Geometry: final body of the model. Coordinates: model frame, mm. Face numbers are marked on the shaded views. A direction names the side the tool comes from. Give positions to 0.01 mm unless a question says otherwise; leave off trailing zeros. Loops run counter-clockwise (first coordinate to the right, second up) from the corner with the lowest first, then second, coordinate; pieces in that order, holes last. Notation, with made-up numbers: M 52,50 L 58,50 A28 ccw 58,75 Z; hole C 42.25,78 d6. An arc over 180 degrees is marked long. Put each result on its own line as item: value.
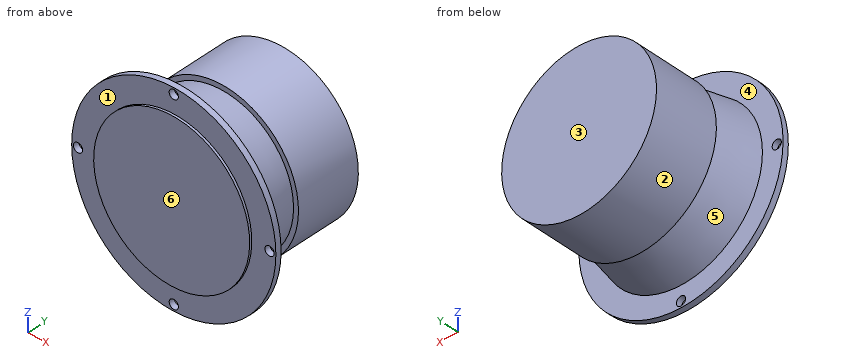
```python
from build123d import *

# Parameters (mm, degrees)
SKETCH1_R           = 44.5
SKETCH1_R_2         = 2
BOSS_EXTRUDE1_DEPTH = 2.5
SKETCH2_R           = 34
BOSS_EXTRUDE2_DEPTH = 1
SKETCH3_R           = 35.5
BOSS_EXTRUDE3_DEPTH = 20
BOSS_EXTRUDE3_TAPER = 11
SKETCH4_R           = 33.75
BOSS_EXTRUDE4_DEPTH = 28.5


with BuildPart() as part:
    # Sketch1 → Boss-Extrude1 (new body)
    with BuildSketch(Plane(origin=(0, 0, 0), x_dir=(1, 0, 0), z_dir=(0, 1, 0))):
        with Locations(Location((0, 0, 0), (0, 0, 270))):
            Circle(SKETCH1_R)
        with Locations(Location((0, 41.75, 0), (0, 0, 270))):
            Circle(SKETCH1_R_2, mode=Mode.SUBTRACT)
        with Locations(Location((41.75, 0, 0), (0, 0, 270))):
            Circle(SKETCH1_R_2, mode=Mode.SUBTRACT)
        with Locations(Location((0, -41.75, 0), (0, 0, 270))):
            Circle(SKETCH1_R_2, mode=Mode.SUBTRACT)
        with Locations(Location((-41.75, 0, 0), (0, 0, 270))):
            Circle(SKETCH1_R_2, mode=Mode.SUBTRACT)
    extrude(amount=BOSS_EXTRUDE1_DEPTH)

    # Sketch2 → Boss-Extrude2 (add)
    with BuildSketch(Plane(origin=(0, 0, 0), x_dir=(-1, 0, 0), z_dir=(0, -1, 0))):
        with Locations(Location((0, 0, 0), (0, 0, 90))):
            Circle(SKETCH2_R)
    extrude(amount=BOSS_EXTRUDE2_DEPTH)

    # Sketch3 → Boss-Extrude3 (add)
    with BuildSketch(Plane(origin=(0, 2.5, 0), x_dir=(1, 0, 0), z_dir=(0, 1, 0))):
        Circle(SKETCH3_R)
    extrude(amount=BOSS_EXTRUDE3_DEPTH, taper=BOSS_EXTRUDE3_TAPER)

    # Sketch4 → Boss-Extrude4 (add)
    with BuildSketch(Plane(origin=(0, 22.5, 0), x_dir=(1, 0, 0), z_dir=(0, 1, 0))):
        with Locations(Location((0, 0, 0), (0, 0, 90))):
            Circle(SKETCH4_R)
    extrude(amount=BOSS_EXTRUDE4_DEPTH)


solid = part.part
```
Item 1: Mould query, pull axis Y, two halves, no side actions, for the marked faces 4, 5 and 6. Classes: pulls with the +Y half, pulls with the -Y half, needs draft (parallel to the pull), parting line crosses it, or undercut.
Output values:
face 4: pulls with the +Y half
face 5: undercut
face 6: pulls with the -Y half
Item 2: Pin query (flat end, axial travel): pin 1 Ø8 at (x, y) = (33, 10) entering from +Z; pin 2 Ø2 at (x, z) = (29.5, 30.5) entering from +Y; pin 3 Ø1.5 at (x, y) = (-2, 14.5) entering from -Z. Return the tip coordinate at first contact, or that it passes through.
Output values:
pin 1: z = 18
pin 2: y = 2.5
pin 3: z = -33.26
Item 3: Section C-C on y = 34. Output: boundary loops of the cut face in (x, z), then the cut area to 3 significant figures.
Output values:
outline: C 0,0 d67.5
area: 3,580 mm²
Item 4: Line query: probe 1 along X at (y, z) = (1.1, 0); probe 2 along X at (y, z) = (1, 41); probe 3 along Y at (x, z) = (26, 35). Output: solid intervals per line, ascending. Write a range as [from, to].
Output values:
probe 1: [-44.5, -43.75], [-39.75, 39.75], [43.75, 44.5]
probe 2: [-17.3, -1.85], [1.85, 17.3]
probe 3: [0, 2.5]
Item 5: Section D-D on x = 0. Output: boundary loops of the cut face in (y, z), then the cut area to 3 significant figures.
Output values:
outline: M -1,-34 L 0,-34 L 0,-39.75 L 2.5,-39.75 L 2.5,-35.5 L 22.5,-31.61 L 22.5,-33.75 L 51,-33.75 L 51,33.75 L 22.5,33.75 L 22.5,31.61 L 2.5,35.5 L 2.5,39.75 L 0,39.75 L 0,34 L -1,34 Z; M 0,-44.5 L 2.5,-44.5 L 2.5,-43.75 L 0,-43.75 Z; M 0,43.75 L 2.5,43.75 L 2.5,44.5 L 0,44.5 Z
area: 3,540 mm²
Item 6: Set-up query: the marked faces 1, 2 and 3. Return all of +Z, -Z, +X, -X, +Y, -Y with unobstructed straight access to the full face (end or side cutting, diameter ignored); none if empty.
Output values:
face 1: -Y
face 2: +Y
face 3: +Z, -Z, +X, -X, +Y
Item 7: Section B-B on x = -41.75. Output: boundary loops of the cut face in (y, z).
Output values:
outline: M 0,-15.4 L 2.5,-15.4 L 2.5,-2 L 0,-2 Z; M 0,2 L 2.5,2 L 2.5,15.4 L 0,15.4 Z
Item 8: Section A-A on z = -41.75. Output: boundary loops of the cut face in (x, y), then the cut area to 3 significant figures.
Output values:
outline: M -15.4,0 L -2,0 L -2,2.5 L -15.4,2.5 Z; M 2,0 L 15.4,0 L 15.4,2.5 L 2,2.5 Z
area: 67.0 mm²
